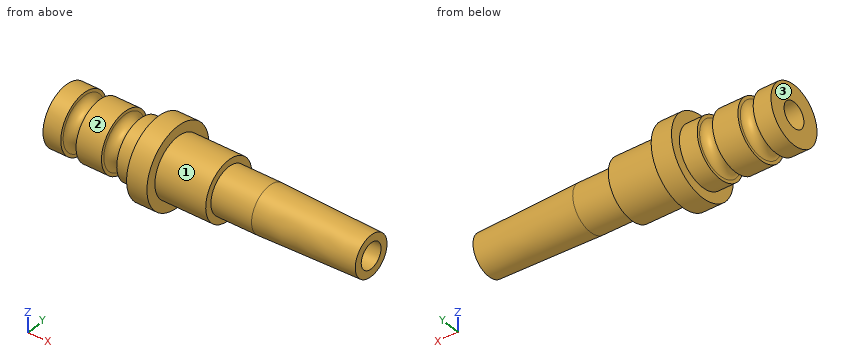
Autodesk Inventor part; units mm, degrees
ref_plane "Work Plane1" through (-22, 0, 2.9) normal (0, 0, 1) x (1, 0, 0)
ref_plane "YZ Plane" through (0, 0, 0) normal (1, 0, 0) x (0, 1, 0)
ref_plane "XZ Plane" through (0, 0, 0) normal (0, 1, 0) x (-1, 0, 0)
sketch "Sketch1" plane through (0, 0, 0) normal (0, 1, 0) x (-1, 0, 0)
  line L0 (0, 0) -> (30, 0)
  line L1 (30, 0) -> (30, -2.9)
  line L2 (30, -2.9) -> (14, -2.9)
  line L3 (0, 0) -> (0, -2)
  line L4 (0, -2) -> (10, -2.25)
  line L5 (14, -2.9) -> (14, -2.25)
  line L6 (10, -2.25) -> (14, -2.25)
  dimension "d0" = 30
  dimension "d1" = 2.9
  dimension "d2" = 16
  dimension "d3" = 2
  dimension "d5" = 4.5
  dimension "d6" = 10
  dimension "d20" = 4
revolve "Revolution1" add sketch "Sketch1" angle 360 about axis through (0, 0, 0) along (-1, 0, 0)
sketch "Sketch2" plane through (0, 0, 0) normal (0, 0, 1) x (1, 0, 0)
  line L0 (-14, -2.9) -> (-14, 2.9) construction
  line L1 (-30, -2.9) -> (-30, 2.9) construction
  line L2 (-30, 2.9) -> (-14, 2.9)
  line L3 (-30, -2.9) -> (-30, 2.9)
  line L4 (-30, 0) -> (0, 0)
  line L5 (-19, 1.9) -> (-19, 3.9)
  line L6 (-19, 3.9) -> (-21, 3.9)
  line L7 (-21, 3.9) -> (-21, 1.9)
  line L8 (-21, 1.9) -> (-19, 1.9)
  line L9 (-30, 2.9) -> (-14, 2.9)
  line L10 (-19, 1.9) -> (-21, 3.9) construction
  line L11 (-19, 3.9) -> (-21, 1.9) construction
  line L12 (-30, 2.9) -> (-14, 2.9)
  point P0 (-20, 2.9)
  dimension "d39" = 2
  dimension "d40" = 1
  dimension "d42" = 5
revolve "Revolution2" add sketch "Sketch2" angle 360 about axis through (-30, 0, 0) along (1, 0, 0)
sketch "Sketch4" plane through (0, 0, 0) normal (1, 0, 0) x (0, 0, -1)
  circle A0 centre (0, 0) radius 1.25
  dimension "d14" = 2.5
extrude "Extrusion1" cut sketch "Sketch4" against normal through all
ref_plane "Work Plane1" through (-22, 0, 2.9) normal (0, 0, 1) x (1, 0, 0)
sketch "Sketch3" plane through (0, 0, 0) normal (0, 0, 1) x (1, 0, 0)
  line L0 (-30, -2.9) -> (-30, 2.9)
  line L1 (-30, 0) -> (0, 0)
  line L2 (-27.5, 3.2) -> (-27.5, 2.6) construction
  line L3 (-30, 2.9) -> (-21, 2.9)
  line L4 (-30, 2.9) -> (-21, 2.9)
  line L5 (-28.25, 3.2) -> (-28.25, 2.6)
  line L6 (-26.75, 2.6) -> (-26.75, 3.2)
  arc A0 (-26.75, 3.2) -> (-28.25, 3.2) centre (-27.5, 3.2) ccw
  arc A1 (-28.25, 2.6) -> (-26.75, 2.6) centre (-27.5, 2.6) ccw
  line L7 (-23.5, 3.2) -> (-23.5, 2.6) construction
  line L8 (-24.25, 3.2) -> (-24.25, 2.6)
  line L9 (-22.75, 2.6) -> (-22.75, 3.2)
  arc A2 (-22.75, 3.2) -> (-24.25, 3.2) centre (-23.5, 3.2) ccw
  arc A3 (-24.25, 2.6) -> (-22.75, 2.6) centre (-23.5, 2.6) ccw
  point P0 (-27.5, 2.9)
  point P1 (-23.5, 2.9)
  dimension "d28" = 1.5
  dimension "d29" = 0.3
  dimension "d30" = 2.5
  dimension "d34" = 4
revolve "Revolution5" cut sketch "Sketch3" angle 360 about axis through (-30, 0, 0) along (1, 0, 0)
properties part number "Connection" material "Nylon 6/6"
CAD build for the part. Positions are in the model's coordinates, mm. Face numbers are marked on the shaded views. A direction names the side the tool comes from. Give positions to 0.01 mm unless a question says otherwise; leave off trailing zeros. Order: outer loops, then holes, each group sorted by start corner. A loop starts at its lowest first (then second) coordinate and runs counter-clockwise, first axis right, second up. Notation, with made-up numbers: M 15,76.25 L 53,76.25 A29 ccw 53,97.25 Z; hole C 82.5,-38 d1. An arc over 180 degrees is marked long. Put each result on its own line as item: value. Start each with the question number.
(1) Which spindle directions (+Z, -Z, +X, -X, +Y, -Y) get a long thin tool onto all of the face, cutting with end or side? Do the marked faces 1, 2 and 3. Say none if no direction does.
(2) Saw through at A-A, the plane x = -25. Write the cut outline in (y, z), then the cut area to 3 significant figures.
(3) Flat gauge pins, fed straight in: pin 1 Ø1 at (x, y) = (-15.5, 0) entering from +Z; pin 2 Ø2 at (x, z) = (-19.5, 2.5) entering from +Y; pin 3 Ø1.5 at (x, z) = (-16, -1) entering from -Y. Where does each tip first touch, or does it go through?
(4) Saw through at B-B, the plane x = -7. Write the cut outline in (y, z) (3 decimals), then the cut area to 3 significant figures.
(5) Drill centre lines: line 1 along X through (y, z) = (2.5, -1); line 2 along Y through (x, z) = (-14.5, 0); line 3 along X through (y, z) = (-2.5, -1.75). Where is each one in solid material? Low to high.
Check result:
1. face 1: +X
1. face 2: -X
1. face 3: +Z, -Z, -X, +Y, -Y
2. outline: C 0,0 d5.8; hole C 0,0 d2.5
2. area: 21.5 mm2
3. pin 1: stops at z = 2.9
3. pin 2: stops at y = 3.6
3. pin 3: stops at y = -2.89
4. outline: C 0,0 d4.35; hole C 0,0 d2.5
4. area: 9.95 mm2
5. line 1: x = -30 to -28.25, -26.75 to -24.25, -22.75 to -14
5. line 2: y = -2.9 to -1.25, 1.25 to 2.9
5. line 3: x = -21 to -19
